Autodesk Inventor part; units mm, degrees
ref_plane "YZ Plane" through (0, 0, 0) normal (1, 0, 0) x (0, 1, 0)
ref_plane "XZ Plane" through (0, 0, 0) normal (0, 1, 0) x (-1, 0, 0)
ref_plane "XY Plane" through (0, 0, 0) normal (0, 0, 1) x (1, 0, 0)
sketch "Gear_Profile_Sketch" plane through (0, 0, 0) normal (0, 0, 1) x (1, 0, 0)
  line L0 (17.4461, -1.373) -> (21.9623, -1.2871)
  line L1 (21.9623, -1.2871) -> (21.8933, 2.1644)
  line L2 (21.8933, 2.1644) -> (17.4461, 1.373)
  line L3 (17.4461, 1.373) -> (17.0165, 4.0853)
  line L4 (17.0165, 4.0853) -> (21.2852, 5.5626)
  line L5 (21.2852, 5.5626) -> (20.1529, 8.8238)
  line L6 (20.1529, 8.8238) -> (16.1679, 6.697)
  line L7 (16.1679, 6.697) -> (14.9212, 9.1437)
  line L8 (14.9212, 9.1437) -> (18.5244, 11.8678)
  line L9 (18.5244, 11.8678) -> (16.4398, 14.6196)
  line L10 (16.4398, 14.6196) -> (13.3071, 11.3653)
  line L11 (13.3071, 11.3653) -> (11.3653, 13.3071)
  line L12 (11.3653, 13.3071) -> (13.9504, 17.0113)
  line L13 (13.9504, 17.0113) -> (11.1175, 18.9842)
  line L14 (11.1175, 18.9842) -> (9.1437, 14.9212)
  line L15 (9.1437, 14.9212) -> (6.697, 16.1679)
  line L16 (6.697, 16.1679) -> (8.0109, 20.4897)
  line L17 (8.0109, 20.4897) -> (4.707, 21.4906)
  line L18 (4.707, 21.4906) -> (4.0853, 17.0165)
  line L19 (4.0853, 17.0165) -> (1.373, 17.4461)
  line L20 (1.373, 17.4461) -> (1.2871, 21.9623)
  line L21 (1.2871, 21.9623) -> (-2.1644, 21.8933)
  line L22 (-2.1644, 21.8933) -> (-1.373, 17.4461)
  line L23 (-1.373, 17.4461) -> (-4.0853, 17.0165)
  line L24 (-4.0853, 17.0165) -> (-5.5626, 21.2852)
  line L25 (-5.5626, 21.2852) -> (-8.8238, 20.1529)
  line L26 (-8.8238, 20.1529) -> (-6.697, 16.1679)
  line L27 (-6.697, 16.1679) -> (-9.1437, 14.9212)
  line L28 (-9.1437, 14.9212) -> (-11.8678, 18.5244)
  line L29 (-11.8678, 18.5244) -> (-14.6196, 16.4398)
  line L30 (-14.6196, 16.4398) -> (-11.3653, 13.3071)
  line L31 (-11.3653, 13.3071) -> (-13.3071, 11.3653)
  line L32 (-13.3071, 11.3653) -> (-17.0113, 13.9504)
  line L33 (-17.0113, 13.9504) -> (-18.9842, 11.1175)
  line L34 (-18.9842, 11.1175) -> (-14.9212, 9.1437)
  line L35 (-14.9212, 9.1437) -> (-16.1679, 6.697)
  line L36 (-16.1679, 6.697) -> (-20.4897, 8.0109)
  line L37 (-20.4897, 8.0109) -> (-21.4906, 4.707)
  line L38 (-21.4906, 4.707) -> (-17.0165, 4.0853)
  line L39 (-17.0165, 4.0853) -> (-17.4461, 1.373)
  line L40 (-17.4461, 1.373) -> (-21.9623, 1.2871)
  line L41 (-21.9623, 1.2871) -> (-21.8933, -2.1644)
  line L42 (-21.8933, -2.1644) -> (-17.4461, -1.373)
  line L43 (-17.4461, -1.373) -> (-17.0165, -4.0853)
  line L44 (-17.0165, -4.0853) -> (-21.2852, -5.5626)
  line L45 (-21.2852, -5.5626) -> (-20.1529, -8.8238)
  line L46 (-20.1529, -8.8238) -> (-16.1679, -6.697)
  line L47 (-16.1679, -6.697) -> (-14.9212, -9.1437)
  line L48 (-14.9212, -9.1437) -> (-18.5244, -11.8678)
  line L49 (-18.5244, -11.8678) -> (-16.4398, -14.6196)
  line L50 (-16.4398, -14.6196) -> (-13.3071, -11.3653)
  line L51 (-13.3071, -11.3653) -> (-11.3653, -13.3071)
  line L52 (-11.3653, -13.3071) -> (-13.9504, -17.0113)
  line L53 (-13.9504, -17.0113) -> (-11.1175, -18.9842)
  line L54 (-11.1175, -18.9842) -> (-9.1437, -14.9212)
  line L55 (-9.1437, -14.9212) -> (-6.697, -16.1679)
  line L56 (-6.697, -16.1679) -> (-8.0109, -20.4897)
  line L57 (-8.0109, -20.4897) -> (-4.707, -21.4906)
  line L58 (-4.707, -21.4906) -> (-4.0853, -17.0165)
  line L59 (-4.0853, -17.0165) -> (-1.373, -17.4461)
  line L60 (-1.373, -17.4461) -> (-1.2871, -21.9623)
  line L61 (-1.2871, -21.9623) -> (2.1644, -21.8933)
  line L62 (2.1644, -21.8933) -> (1.373, -17.4461)
  line L63 (1.373, -17.4461) -> (4.0853, -17.0165)
  line L64 (4.0853, -17.0165) -> (5.5626, -21.2852)
  line L65 (5.5626, -21.2852) -> (8.8238, -20.1529)
  line L66 (8.8238, -20.1529) -> (6.697, -16.1679)
  line L67 (6.697, -16.1679) -> (9.1437, -14.9212)
  line L68 (9.1437, -14.9212) -> (11.8678, -18.5244)
  line L69 (11.8678, -18.5244) -> (14.6196, -16.4398)
  line L70 (14.6196, -16.4398) -> (11.3653, -13.3071)
  line L71 (11.3653, -13.3071) -> (13.3071, -11.3653)
  line L72 (13.3071, -11.3653) -> (17.0113, -13.9504)
  line L73 (17.0113, -13.9504) -> (18.9842, -11.1175)
  line L74 (18.9842, -11.1175) -> (14.9212, -9.1437)
  line L75 (14.9212, -9.1437) -> (16.1679, -6.697)
  line L76 (16.1679, -6.697) -> (20.4897, -8.0109)
  line L77 (20.4897, -8.0109) -> (21.4906, -4.707)
  line L78 (21.4906, -4.707) -> (17.0165, -4.0853)
  line L79 (17.0165, -4.0853) -> (17.4461, -1.373)
extrude "Extrusion1" add sketch "Gear_Profile_Sketch" against normal blind 13.86
properties part number "pinn_optimized_geometry"
Can you work these out from the model? Positions are in its coordinate system, mm. A direction names the side the tool comes from. Coordinates: 2 decimals unless noted, no trailing zeros. Order: outer loops, then holes, each group sorted by start corner. A loop starts at its lowest first (then second) coordinate and runs counter-clockwise, first axis right, second up.
1. I'm going to push flat-ended pins straight in: pin 1 (1.5 mm diameter, centred on x = 15, y = 6.5, fed in from +Z); pin 2 (8 mm diameter, centred on y = -11.5, z = -4, fed in from -X); pin 3 (1 mm diameter, centred on y = 9, z = -2.5, fed in from +X). Where does each tip first touch, or does it pass through?
2. If we section it at A-A (y = 15.5): Please give me the cut outline in (x, z).
3. If we section it at B-B (x = 3): Please give me the cut outline in (y, z), then the cut area to 3 significant figures.
4. I need wall thicknesses on line 1 (X direction, y = -20, z = -12); line 2 (Y direction, x = -17.5, z = -3); line 3 (Y direction, x = 13, z = -3.5). Which ranges of each line are inside material? Lowest first, please.
5. Thinking about a two-plate mould opening in Y: for faces 4 (the face through (6.382, 20.983, -6.833)), 5 (the face through (-6.382, -20.983, -6.833)), 6 (the face through (-17.23, 2.75, -6.83)), which applies, +Y half, -Y half, draft (parallel to the pull), parting line (faces both ways), or undercut?
6. For faces 1 (the face through (7.17, -20.727, -6.833)), 2 (the face through (-4.814, 19.121, -6.833)), 3 (the face through (-17.234, -2.71, -6.833)), which set-ups out of +Z, -Z, +X, -X, +Y, -Y let a thin tool reach every point of the face, with its end or its side?
Entries:
1. pin 1: stops at z = 0
1. pin 2: stops at x = -20.61
1. pin 3: stops at x = 20.27
2. outline: (-13.64, -13.86) - (-9.58, -13.86) - (-9.58, 0) - (-13.64, 0) - close; (-8.01, -13.86) - (8.01, -13.86) - (8.01, 0) - (-8.01, 0) - close; (9.42, -13.86) - (12.9, -13.86) - (12.9, 0) - (9.42, 0) - close
3. outline: (-17.19, -13.86) - (17.19, -13.86) - (17.19, 0) - (-17.19, 0) - close
3. area: 476 mm2
4. line 1: x = -7.86 to -4.5, -1.32 to 1.83, 5.12 to 8.74
4. line 2: y = -13.22 to -11.09, -7.41 to -4.25, -1.38 to 1.37, 4.15 to 7.1, 10.4 to 13.25
4. line 3: y = -17.67 to -14.88, -11.67 to 11.67, 15.65 to 17.67
5. face 4: +Y half
5. face 5: -Y half
5. face 6: undercut
6. face 1: +Z, -Z, +X, -Y
6. face 2: +Z, -Z, +Y
6. face 3: +Z, -Z
